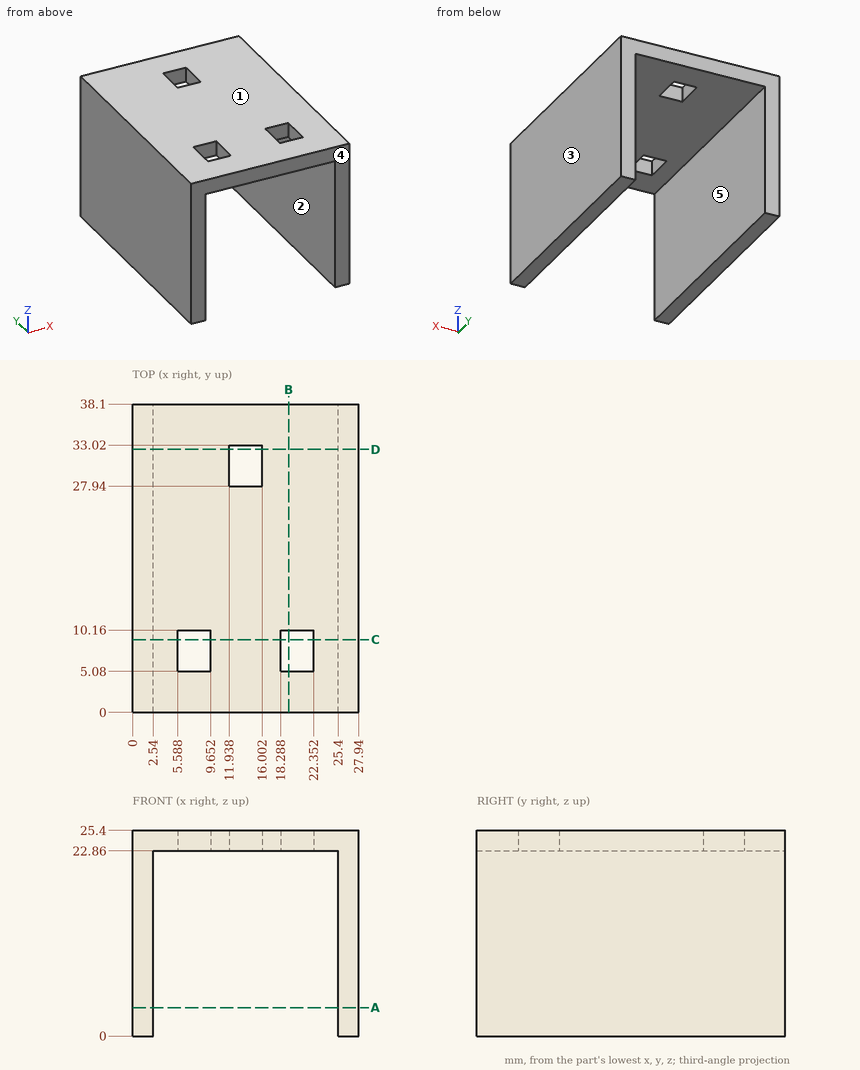
Answer from the drawing. Dimensions are ordinates in mm from the lowest x, y and z of the part. A direction names the side the tool comes from. Coordinates: 2 decimals unless noted, no trailing zeros. Write each loop counter-clockwise with the first axis right and the second up, starting at its lowest first coordinate (ties: lowest second). Pieces come first, ordered by that corner, then holes. Notation, with made-up numbers: (87.25, -25) - (120.25, -25) arc R12 cw to (120.25, -14) - close; hole circle Ø10 at (2, -14). An arc over 180 degrees is marked (long way). Return JSON: item names as keys, results as strings. Group by question number.
Q1. For a pull along X with two mould halves and no side action, classify the marked faces 3, 4 and 5 as +X half, -X half, draft (parallel to the pull), parting line (faces both ways), or undercut.
Q2. The part is cut by section C-C on y = 9. Write down the section's boundary in (x, z), and give its area (3 significant figures).
Q3. Flat-ended cylindrical pins translate along their axes: pin 1 Ø7 at (x, y) = (13.5, 15) entering from -Z; pin 2 Ø12 at (x, z) = (12.5, 4.5) entering from -Y. Find the tip coordinate at first contact, or state that the pin passes through.
Q4. The part is cut by section B-B on x = 19.25. Write down the section's boundary in (y, z).
Q5. Which of the six approach directions +Z, -Z, +X, -X, +Y, -Y give full straight-line access (tool end or side, diameter ignored) to the marked faces 1 and 2?
Q6. The part is cut by section A-A on z = 3.5. Write down the section's boundary in (x, y).
Q7. Find the intervals of material crossed by line 1 along X through (y, z) = (34.5, 18.25); line 2 along Z through (x, y) = (17.75, 3), in increasing order. Write a range as [from, to].
Q8. The part is cut by section D-D on y = 32.5. Write down the section's boundary in (x, z), and give its area (3 significant figures).
Evaluation:
{
 "1": {"face 3": "+X half", "face 4": "draft", "face 5": "undercut"},
 "2": {"outline": "(0, 0) - (2.54, 0) - (2.54, 22.86) - (5.59, 22.86) - (5.59, 25.4) - (0, 25.4) - close; (9.65, 22.86) - (18.29, 22.86) - (18.29, 25.4) - (9.65, 25.4) - close; (22.35, 22.86) - (25.4, 22.86) - (25.4, 0) - (27.94, 0) - (27.94, 25.4) - (22.35, 25.4) - close", "area": "166 mm2"},
 "3": {"pin 1": "stops at z = 22.86", "pin 2": "passes through"},
 "4": {"outline": "(0, 22.86) - (5.08, 22.86) - (5.08, 25.4) - (0, 25.4) - close; (10.16, 22.86) - (38.1, 22.86) - (38.1, 25.4) - (10.16, 25.4) - close"},
 "5": {"face 1": "+Z, +X, -X, +Y, -Y", "face 2": "-Z, +Y, -Y"},
 "6": {"outline": "(0, 0) - (2.54, 0) - (2.54, 38.1) - (0, 38.1) - close; (25.4, 0) - (27.94, 0) - (27.94, 38.1) - (25.4, 38.1) - close"},
 "7": {"line 1": "x = [0, 2.54], [25.4, 27.94]", "line 2": "z = [22.86, 25.4]"},
 "8": {"outline": "(0, 0) - (2.54, 0) - (2.54, 22.86) - (11.94, 22.86) - (11.94, 25.4) - (0, 25.4) - close; (16, 22.86) - (25.4, 22.86) - (25.4, 0) - (27.94, 0) - (27.94, 25.4) - (16, 25.4) - close", "area": "177 mm2"}
}
